```python
from build123d import *

# Parameters (mm, degrees)
F1_DEPTH = 28
F2_R     = 1.5
F3_DEPTH = 5
F4_R     = 1.5
F5_DEPTH = 3


with BuildPart() as f1:
    # F0 (on Top) → F1 (new body)
    with BuildSketch(Plane.XY):
        Polygon((-1.028917, 3.488743), (-3.535799, 0.853303), (-2.506882, -2.63544), (1.028917, -3.488743), (3.535799, -0.853303), (2.506882, 2.63544), align=None)
    extrude(amount=F1_DEPTH)

    # F2 (on face) → F3 (join)
    with BuildSketch(Plane.XY.offset(28)):
        Circle(F2_R)
    extrude(amount=F3_DEPTH)

    # F4 (on face) → F5 (join)
    with BuildSketch(Plane(origin=(0, 0, 0), x_dir=(1, 0, 0), z_dir=(0, 0, -1))):
        Circle(F4_R)
    extrude(amount=F5_DEPTH)


solid = f1.part
```
CAD build for the part. Positions are in the model's coordinates, mm. A direction names the side the tool comes from. Round coordinates to 2 decimals unless told otherwise and drop trailing zeros. Order: outer loops, then holes, each group sorted by start corner. A loop starts at its lowest first (then second) coordinate and runs counter-clockwise, first axis right, second up.
Item 1: Probe line 1 along Z through (x, y) = (-2, -2.25); line 2 along X through (y, z) = (0, 20.5); line 3 along X through (y, z) = (0.5, 30.5). List the from-to ranges inside material, lowest first.
Item 2: Saw through at D-D on x = -2. Write the cut outline in (y, z), then the cut area to 3 significant figures.
Item 3: Saw through at A-A on x = -0.25. Write the cut outline in (y, z).
Item 4: Saw through at B-B on y = 0. Write the cut outline in (x, z), then the cut area to 3 significant figures.
Item 5: Pin check, flat tips, straight feed: pin 1 (3 mm diameter, centred on y = 2.5, z = 23, fed in from -X); pin 2 (1.5 mm diameter, centred on x = -2.5, y = -2, fed in from -Z). Stop position of each tip, or through.
Item 6: Tool access for faces 1 (the face through (2.265, -2.189, 13.804)), 2 (the face through (-1.5, 0.07, 30.46)), 3 (the face through (-1.5, -0.07, -1.48)): list every direction of +Z, -Z, +X, -X, +Y, -Y with a clear straight run to the whole face (end or side of a thin tool).
Item 7: Saw through at C-C on z = 14. Write the cut outline in (x, y).
Reported:
1. line 1: z = 0 to 28
1. line 2: x = -3.28 to 3.28
1. line 3: x = -1.41 to 1.41
2. outline: (-2.76, 0) - (2.47, 0) - (2.47, 28) - (-2.76, 28) - close
2. area: 146 mm2
3. outline: (-3.18, 0) - (-1.48, 0) - (-1.48, -3) - (1.48, -3) - (1.48, 0) - (3.3, 0) - (3.3, 28) - (1.48, 28) - (1.48, 33) - (-1.48, 33) - (-1.48, 28) - (-3.18, 28) - close
4. outline: (-3.28, 0) - (-1.5, 0) - (-1.5, -3) - (1.5, -3) - (1.5, 0) - (3.28, 0) - (3.28, 28) - (1.5, 28) - (1.5, 33) - (-1.5, 33) - (-1.5, 28) - (-3.28, 28) - close
4. area: 208 mm2
5. pin 1: stops at x = -3.4
5. pin 2: stops at z = 0
6. face 1: +Z, -Z, +X, -Y
6. face 2: +Z
6. face 3: -Z
7. outline: (-3.54, 0.85) - (-2.51, -2.64) - (1.03, -3.49) - (3.54, -0.85) - (2.51, 2.64) - (-1.03, 3.49) - close
